Autodesk Inventor part; units mm, degrees
ref_plane "YZ Plane" through (0, 0, 0) normal (1, 0, 0) x (0, 1, 0)
ref_plane "XZ Plane" through (0, 0, 0) normal (0, 1, 0) x (-1, 0, 0)
ref_plane "XY Plane" through (0, 0, 0) normal (0, 0, 1) x (1, 0, 0)
sketch "スケッチ1" plane through (0, 0, 0) normal (0, 1, 0) x (-1, 0, 0)
  line L0 (0, 0) -> (-220, 0)
  line L1 (-220, 0) -> (-220, -35)
  line L2 (-220, -35) -> (0, -35)
  line L3 (0, -35) -> (0, 0)
  arc A0 (0, -35) -> (0, 0) centre (0, -17.5) ccw
  dimension "d0" = 220
  dimension "d1" = 35
  dimension "d2" = 17.5
extrude "押し出し1" add sketch "スケッチ1" along normal blind 3
sketch "スケッチ2" plane through (0, 3, 0) normal (0, 1, 0) x (1, 0, 0)
  line L0 (0, 17.5) -> (238.6526, 17.5)
  line L1 (0, 0) -> (220, 0)
  arc A0 (0, 35) -> (0, 0) centre (0, 17.5) ccw
  point P0 (20, 17.5)
  point P1 (30, 17.5)
  point P2 (40, 17.5)
  point P3 (50, 17.5)
  point P4 (60, 17.5)
  point P5 (70, 17.5)
  point P6 (80, 17.5)
  point P7 (90, 17.5)
  point P8 (100, 17.5)
  point P9 (110, 17.5)
  point P10 (120, 17.5)
  point P11 (130, 17.5)
  point P12 (140, 17.5)
  point P13 (150, 17.5)
  point P14 (160, 17.5)
  point P15 (170, 17.5)
  point P16 (180, 17.5)
  point P17 (190, 17.5)
  point P18 (200, 17.5)
  point P19 (210, 17.5)
  point P20 (-17.5, 17.5)
  point P21 (10, 17.5)
  dimension "d5" = 17.5
  dimension "d6" = 10
  dimension "d7" = 10
  dimension "d8" = 10
  dimension "d9" = 10
  dimension "d10" = 10
  dimension "d11" = 10
  dimension "d12" = 10
  dimension "d13" = 10
  dimension "d14" = 10
  dimension "d15" = 10
  dimension "d16" = 10
  dimension "d17" = 10
  dimension "d18" = 10
  dimension "d19" = 10
  dimension "d20" = 10
  dimension "d21" = 10
  dimension "d22" = 10
  dimension "d23" = 10
  dimension "d24" = 10
  dimension "d35" = 17.5
  dimension "d55" = 10
  dimension "d56" = 10
hole "穴1" at (20, 3, -17.5) at (30, 3, -17.5) at (40, 3, -17.5) at (50, 3, -17.5) at (60, 3, -17.5) at (70, 3, -17.5) at (80, 3, -17.5) at (90, 3, -17.5) at (100, 3, -17.5) at (110, 3, -17.5) at (120, 3, -17.5) at (130, 3, -17.5) at (140, 3, -17.5) at (150, 3, -17.5) at (160, 3, -17.5) at (170, 3, -17.5) at (180, 3, -17.5) at (190, 3, -17.5) at (200, 3, -17.5) at (210, 3, -17.5) at (10, 3, -17.5) direction (0, -1, 0) diameter 3.2 end through all
sketch "スケッチ3" plane through (0, 3, 0) normal (0, 1, 0) x (1, 0, 0)
  line L0 (220, 35) -> (0, 35)
  point P0 (0, 0)
  point P1 (0, 17.5)
  dimension "d36" = 17.5
hole "穴2" [suppressed]
sketch "スケッチ4" plane through (0, 3, 0) normal (0, 1, 0) x (1, 0, 0)
  circle A0 centre (0, 17.5) radius 6
  circle A1 centre (0, 17.5) radius 3.15
  line L0 (-0.1439, 17.5) -> (-6.5454, 17.5)
  line L1 (-6.5454, 17.5) -> (7.5104, 17.5)
  point P0 (0, 0)
  point P1 (0, 11.5)
  point P2 (6, 17.5)
  point P3 (0, 23.5)
  point P4 (-6, 17.5)
  dimension "d44" = 12
  dimension "d45" = 0
hole "穴3" [suppressed]
properties part number "arm_plate4" material "アルミニウム 5052"
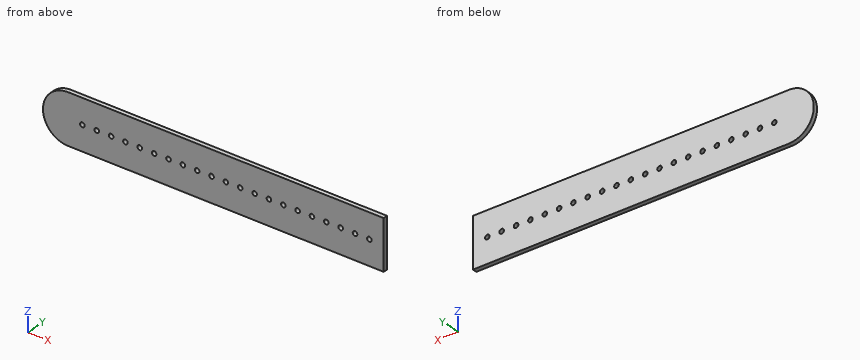
Can you work these out from the model? Positions are in its coordinate system, mm. Give positions to 0.01 mm unless a question says otherwise; leave off trailing zeros. Order: outer loops, then holes, each group sorted by start corner. A loop starts at its lowest first (then second) coordinate and runs counter-clockwise, first axis right, second up. Notation, with made-up numbers: M 63,76 L 88,76 A24 cw 88,89 Z; hole C 58.25,87 d8. An arc over 180 degrees is marked long. Use one line per item in the form item = value. Start each with the question number.
Item 1: If we section it at A-A (y = 2.2): State how many separate pieces and enclosed holes the cut face has, then the cut area to 3 significant figures.
Item 2: Will this pin go through, and if not, where does the flat tip stop? pin 1 Ø1.9 at (x, z) = (80, -17.5) entering from +Y.
Item 3: If I drill on line 1 along Z through (x, y) = (100, 1); line 2 along X through (y, z) = (1.85, -22.5); line 3 along X through (y, z) = (2.5, -29), over which ranges is the centre line in solid material (lowest first)?
Item 4: If we section it at B-B (z = -31.5): Write out the boundary of the cut face in (x, y).
Outcome:
q1.separate_pieces = 1
q1.enclosed_holes = 21
q1.area = 8,010 mm2
q2.pin_1 = through
q3.line_1 = -35 to -19.1, -15.9 to 0
q3.line_2 = -16.77 to 220
q3.line_3 = -13.19 to 220
q4.outline = M -10.5,0 L 220,0 L 220,3 L -10.5,3 Z
